The listing builds one solid part. Answer for the finished solid, in the listing's coordinates (mm). Face numbers are marked on the shaded views. A direction names the side the tool comes from. Give positions to 0.01 mm unless a question says otherwise; leave off trailing zeros. Write each loop counter-clockwise with the first axis right and the second up, starting at its lowest first coordinate (ties: lowest second). Pieces come first, ordered by that corner, then holes. Notation, with made-up numbers: (-37.5, 68.25) - (-2.5, 68.25) arc R31 cw to (-2.5, 100.25) - close; hole circle Ø7 at (-26.5, 61). An arc over 180 degrees is marked (long way). Answer as CSV lines item,"result". Start each with the question number.
(1) Straight lines are drawn through the part: probe 1 along Y at (x, z) = (10.75, -67.5); probe 2 along Y at (x, z) = (7, -74); probe 3 along Z at (x, y) = (1.5, -47.5). For each, find the intervals that lie inside material, in ascending order.
(2) For a pull along Y with two mould halves and no side action, classify the marked faces 4, 5 and 6 as pulls with the +Y half, pulls with the -Y half, needs draft (parallel to the pull), parting line crosses it, or undercut.
(3) Each of these flat-tipped pins is pushed along its axis until it touches: pin 1 Ø1.5 at (x, z) = (9.5, -65) entering from -Y; pin 2 Ø2 at (x, z) = (11.5, -90) entering from -Y; pin 3 Ø1.5 at (x, z) = (11.5, -49) entering from -Y. Where does it stop, or does it pass through?
(4) For the marked faces 1, 2 and 3, determine the directions among +Z, -Z, +X, -X, +Y, -Y from which every point of the face is accessible in a straight line to the end or side of a thin tool.
(5) Find section A-A (z = -53.5). Write down the section's boundary in (x, y).
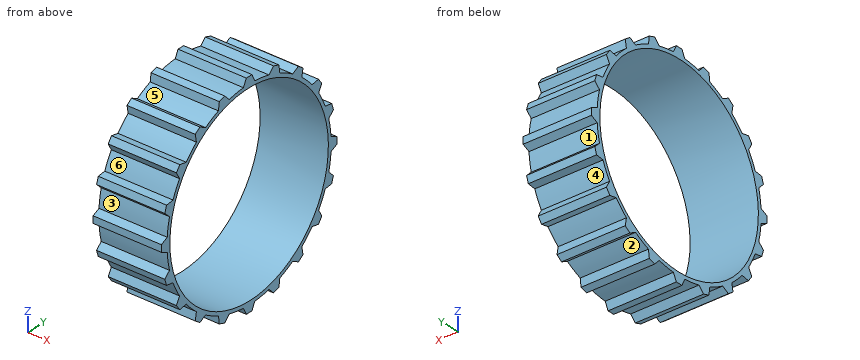
from build123d import *

# Parameters (mm, degrees)
SKETCH1_R           = 29
SKETCH1_R_2         = 28
BOSS_EXTRUDE1_DEPTH = 20
BOSS_EXTRUDE2_DEPTH = 20
CIRPATTERN1_COUNT   = 20


with BuildPart() as part:
    # Sketch1 → Boss-Extrude1 (new body)
    with BuildSketch(Plane(origin=(13.876749841, 0, 0), x_dir=(0, 0, -1), z_dir=(1, 0, 0))):
        with Locations((67.469370674, -50.661515593)):
            Circle(SKETCH1_R)
        with Locations((67.469370674, -50.661515593)):
            Circle(SKETCH1_R_2, mode=Mode.SUBTRACT)
    extrude(amount=-BOSS_EXTRUDE1_DEPTH)

    # Sketch2 → Boss-Extrude2 (add, through all)
    with BuildSketch(Plane(origin=(13.876749841, 0, 0), x_dir=(0, 0, -1), z_dir=(1, 0, 0))):
        with BuildLine():
            Line((66.469370674, -19.661515593), (65.469370674, -21.73056331))
            ThreePointArc((65.469370674, -21.73056331), (67.469370674, -21.661515593), (69.469370674, -21.73056331))
            Line((69.469370674, -21.73056331), (68.469370674, -19.661515593))
            Line((68.469370674, -19.661515593), (66.469370674, -19.661515593))
        make_face()
    boss_extrude2 = extrude(amount=-BOSS_EXTRUDE2_DEPTH)

    # CirPattern1: Boss-Extrude2 ×20 about axis
    cirpattern1_axis = Axis((0, -50.661515593, -67.469370674), (1, 0, 0))
    for i in range(1, CIRPATTERN1_COUNT):
        add(boss_extrude2.rotate(cirpattern1_axis, i * 360 / CIRPATTERN1_COUNT))


solid = part.part
Result set:
1,probe 1,"-81.66 to -78.66, -22.66 to -19.66"
1,probe 2,"-78.92 to -77.89, -23.43 to -22.41"
1,probe 3,"-96.3 to -95.29, -39.65 to -38.64"
2,face 4,"pulls with the +Y half"
2,face 5,"undercut"
2,face 6,"pulls with the -Y half"
3,pin 1,"y = -80.17"
3,pin 2,"y = -70.09"
3,pin 3,"y = -76.11"
4,face 1,"+X, -X, +Y"
4,face 2,"-Z, +X, -X"
4,face 3,"+X, -X, -Y"
5,outline,"(-6.12, -76.08) - (13.88, -76.08) - (13.88, -74.93) - (-6.12, -74.93) - close; (-6.12, -26.4) - (13.88, -26.4) - (13.88, -25.25) - (-6.12, -25.25) - close"
